Build history of the part. All positions in model axes, mm. A direction names the side the tool comes from. Round coordinates to 2 decimals unless told otherwise and drop trailing zeros. Write each loop counter-clockwise with the first axis right and the second up, starting at its lowest first coordinate (ties: lowest second). Pieces come first, ordered by that corner, then holes. Notation, with made-up numbers: (16.5, 89.5) -> (72.5, 89.5) arc R28 cw to (72.5, 128.5) -> close; hole circle Ø2 at (53.5, 66.5). An arc over 180 degrees is marked (long way). Answer in a Markdown table with one row per item.
```python
from build123d import *

# Parameters (mm, degrees)
F0_R     = 151
F1_DEPTH = 500
F2_R     = 149
F3_DEPTH = 490
F4_R     = 169
F4_R_2   = 149
F5_DEPTH = 4
F6_R     = 5
F7_DEPTH = 504.001


with BuildPart() as f1:
    # F0 (on Top) → F1 (new body)
    with BuildSketch(Plane.XY):
        Circle(F0_R)
    extrude(amount=F1_DEPTH)

    # F2 (on face) → F3 (cut)
    with BuildSketch(Plane.XY.offset(500)):
        Circle(F2_R)
    extrude(amount=-F3_DEPTH, mode=Mode.SUBTRACT)

    # F4 (on face) → F5 (join)
    with BuildSketch(Plane.XY.offset(500)):
        Circle(F4_R)
        Circle(F4_R_2, mode=Mode.SUBTRACT)
    extrude(amount=F5_DEPTH)

    # F6 (on face) → F7 (cut, through all)
    with BuildSketch(Plane.XY.offset(504)):
        with Locations((0, 161)):
            Circle(F6_R)
        with Locations((-153.120099, 49.751736)):
            Circle(F6_R)
        with Locations((-94.633426, -130.251736)):
            Circle(F6_R)
        with Locations((94.633426, -130.251736)):
            Circle(F6_R)
        with Locations((153.120099, 49.751736)):
            Circle(F6_R)
    extrude(amount=-F7_DEPTH, mode=Mode.SUBTRACT)


solid = f1.part
```
Q1. Drop flat-ended pins along their axis: P1, Ø12, axis at x = 126.5, y = -26, coming from the +Z side; P2, Ø1.5, axis at y = 25.5, z = 56, coming from the -X side; P3, Ø6, axis at x = -153.12, y = 49.75, coming from the -Z side; P4, Ø1.5, axis at y = 54, z = 385.5, coming from the +X side. Give the stop position or say it passes through.
A:
| item | result |
|---|---|
| P1 | z = 10 |
| P2 | x = -148.96 |
| P3 | through |
| P4 | x = 141.3 |
Q2. Saw through at B-B on x = 125. Write the cut outline in (y, z), plus the area to 3 significant figures.
A:
| item | result |
|---|---|
| outline | (-113.74, 500) -> (-84.71, 500) -> (-84.71, 0) -> (84.71, 0) -> (84.71, 500) -> (113.74, 500) -> (113.74, 504) -> (81.09, 504) -> (81.09, 10) -> (-81.09, 10) -> (-81.09, 504) -> (-113.74, 504) -> close |
| area | 5,500 mm² |
Q3. Saw through at A-A on y = 0. Write the cut outline in (x, z).
A:
| item | result |
|---|---|
| outline | (-169, 500) -> (-151, 500) -> (-151, 0) -> (151, 0) -> (151, 500) -> (169, 500) -> (169, 504) -> (149, 504) -> (149, 10) -> (-149, 10) -> (-149, 504) -> (-169, 504) -> close |
Q4. Two-plate mould, pull along X, no slides. Class faces 1 (the cylindrical face through (144.027, 45.356, 246.5)), 2 (the flat face through (99, -112, 504)), 3 (the flat face through (-2, 2, 10)), 4 (the cylindrical face through (142.12, 44.76, 253.54)): released by +X, released by -X, zero draft, split by the parting line, or undercut.
A:
| item | result |
|---|---|
| face 1 | split by the parting line |
| face 2 | zero draft |
| face 3 | undercut |
| face 4 | undercut |
Q5. Which spindle directions (+Z, -Z, +X, -X, +Y, -Y) get a long thin tool onto all of the face, cutting with end or side? Do faces 5 (the flat face through (-138, -62, 500)), 6 (the cylindrical face through (-124.56, 114.22, 501.97)). Say none if no direction does.
A:
| item | result |
|---|---|
| face 5 | -Z |
| face 6 | +Z, -Z |
Q6. Saw through at C-C on z = 312.5. Write the cut outline in (x, y), plus the area to 3 significant figures.
A:
| item | result |
|---|---|
| outline | circle Ø302 at (0, 0); hole circle Ø298 at (0, 0) |
| area | 1,880 mm² |
Q7. Wall check: line 1 (Z direction, x = -117.5, y = -73); line 2 (X direction, y = 4, z = 168); line 3 (Y direction, x = -107, z = 77). Give the ranges that are in metal, low to high. Write a range as [from, to].
A:
| item | result |
|---|---|
| line 1 | [0, 10] |
| line 2 | [-150.95, -148.95], [148.95, 150.95] |
| line 3 | [-106.55, -103.69], [103.69, 106.55] |
